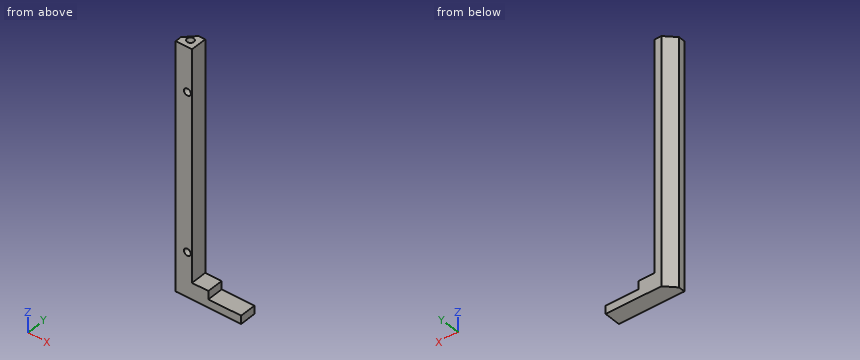
```python
from build123d import *

# Parameters (mm, degrees)
DODANIE_WYCI_GNI_CIE1_DEPTH = 10
SZKIC2_R                    = 2.1
WYTNIJ_WYCI_GNI_CIE1_DEPTH  = 4
SZKIC3_R                    = 2.1
WYTNIJ_WYCI_GNI_CIE2_DEPTH  = 4
SFAZOWANIE1_SIZE            = 6


with BuildPart() as part:
    # Szkic1 → Dodanie-wyciągnięcie1 (new body)
    with BuildSketch(Plane(origin=(0, 0, 0), x_dir=(1, 0, 0), z_dir=(0, 1, 0))):
        Polygon((0, 0), (0, 150), (40, 150), (40, 145), (20, 145), (20, 140), (10, 140), (10, 0), align=None)
    extrude(amount=DODANIE_WYCI_GNI_CIE1_DEPTH)

    # Szkic2 → Wytnij-wyciągnięcie1 (cut)
    with BuildSketch(Plane.XZ):
        with Locations(Location((7.2, -27, 0), (0, 0, 270))):
            Circle(SZKIC2_R)
        with Locations(Location((7.2, -123, 0), (0, 0, 270))):
            Circle(SZKIC2_R)
    extrude(amount=-WYTNIJ_WYCI_GNI_CIE1_DEPTH, mode=Mode.SUBTRACT)

    # Szkic3 → Wytnij-wyciągnięcie2 (cut)
    with BuildSketch(Plane.XY):
        with Locations((5, 5)):
            Circle(SZKIC3_R)
    extrude(amount=-WYTNIJ_WYCI_GNI_CIE2_DEPTH, mode=Mode.SUBTRACT)

    # Sfazowanie1
    sfazowanie1_edges = [part.edges().sort_by_distance(p)[0] for p in [
        (0, 10, -75),
    ]]
    chamfer(sfazowanie1_edges, length=SFAZOWANIE1_SIZE)


solid = part.part
```
Work out the finished part from the listing and answer in its coordinate system (mm). Round coordinates to 2 decimals unless told otherwise and drop trailing zeros. Loops run counter-clockwise (first coordinate to the right, second up) from the corner with the lowest first, then second, coordinate; pieces in that order, holes last.
(1) Each of these flat-tipped pins is pushed along its axis until it touches: P1, Ø1.3, axis at x = 7.5, z = -28, coming from the -Y side; P2, Ø1, axis at x = 14, y = 3.5, coming from the +Z side; P3, Ø1.5, axis at y = 9, z = -53, coming from the +X side; P4, Ø2, axis at x = 4, y = 6, coming from the +Z side. Where does it stop, or does it pass through?
Computed values:
P1: stops at y = 4
P2: stops at z = -140
P3: stops at x = 10
P4: stops at z = 0
(2) The part is cut by section C-C, the plane y = 8.75. Give the vertices of the cut face in (x, z).
Computed values:
outline: (4.75, -150) - (40, -150) - (40, -145) - (20, -145) - (20, -140) - (10, -140) - (10, 0) - (4.75, 0) - close
(3) Find the intervals of material crossed by L1, parallel to X at y = 1.3, z = -123; L2, parallel to Z at x = 32.5, y = 6.5; L3, parallel to X at y = 3.25, z = -53.5, in increasing order.
Computed values:
L1: x = 0 to 5.1, 9.3 to 10
L2: z = -150 to -145
L3: x = 0 to 10
(4) The part is cut by section D-D, the plane x = 29.5. Give the vertices of the cut face in (y, z), and give its area (3 significant figures).
Computed values:
outline: (0, -150) - (10, -150) - (10, -145) - (0, -145) - close
area: 50.0 mm2
(5) The part is cut by section B-B, the plane z = -27. Give the vertices of the cut face in (x, y).
Computed values:
outline: (0, 0) - (5.1, 0) - (5.1, 4) - (9.3, 4) - (9.3, 0) - (10, 0) - (10, 10) - (6, 10) - (0, 4) - close
(6) The part is cut by section A-A, the plane y = 1.5. Give the vertices of the cut face in (x, z), and give its area (3 significant figures).
Computed values:
outline: (0, -150) - (40, -150) - (40, -145) - (20, -145) - (20, -140) - (10, -140) - (10, 0) - (0, 0) - close; hole circle Ø4.2 at (7.2, -123); hole circle Ø4.2 at (7.2, -27)
area: 1,670 mm2
